Autodesk Fusion 360 part; units mm, degrees
sketch "Sketch1" plane through (0, 0, 0) normal (0, 1, 0) x (1, 0, 0)
  line L0 (-33.0001, 0) -> (-35.8285, -2.8284)
  line L1 (-33.0001, 0) -> (-33.002, 0) construction
  line L2 (-35.8285, -2.8284) -> (-35.8285, -23.8284)
  line L3 (-31.8323, -27.8284) -> (-31.8323, -32.0026)
  line L4 (-31.8323, -32.0026) -> (-59.8323, -32.0026)
  line L5 (-59.8323, -32.0026) -> (-59.8323, -48.0026)
  line L6 (-59.8323, -48.0026) -> (-31.8285, -48.0026)
  line L7 (-31.8285, -48.0026) -> (-31.8285, -50.0026)
  line L8 (-35.8285, -54.0026) -> (-35.8285, -75.0026)
  line L9 (-35.8285, -75.0026) -> (-33.0001, -77.8311)
  line L10 (-33.0001, -77.8311) -> (-1.0001, -77.8311)
  line L11 (-33.002, 0) -> (-1.002, 0)
  arc A0 (-35.8285, -54.0026) -> (-31.8285, -50.0026) centre (-35.8285, -50.0026) ccw
  arc A1 (-31.8323, -27.8284) -> (-35.8285, -23.8284) centre (-35.8323, -27.8284) ccw
  line L12 (-1.0001, -77.8311) -> (-1.002, 0)
  point P0 (-31.8323, -24.0026)
  point P1 (-31.8285, -54.0026)
  point P2 (-4.832, 0)
  dimension "d2" = 135
  dimension "d3" = 4
  dimension "d4" = 21
  dimension "d5" = 4
  dimension "d6" = 8
  dimension "d7" = 28
  dimension "d8" = 16
  dimension "d9" = 6
  dimension "d10" = 4
  dimension "d11" = 21
  dimension "d12" = 4
  dimension "d13" = 135
  dimension "d14" = 32
  dimension "d15" = 32
  dimension "d16" = 4
  dimension "d17" = 4
revolve "Revolve1" add sketch "Sketch1" angle 360 about axis through (0, 0, 1.75) along (0, 0, 1)
sketch "Sketch2" plane through (0, 0, 77.8311) normal (0, 0, 1) x (-1, 0, 0)
  circle A0 centre (0, 0) radius 1.0001
  circle A1 centre (0, 0) radius 33.0001
  circle A2 centre (0, 0) radius 24
  dimension "d19" = 48
extrude "Extrude1" cut sketch "Sketch2" against normal blind 110 contours A2
sketch "Sketch3" plane through (0, 0, 48.0026) normal (0, 0, 1) x (-1, 0, 0)
  circle A0 centre (0, 0) radius 31.8285
  circle A1 centre (0, 0) radius 59.8323
  circle A2 centre (0, 0) radius 54
  circle A3 centre (53.999, -0.3261) radius 4
  line L0 (0, 0) -> (27, -46.7654)
  line L1 (0, 0) -> (54, 0) construction
  circle A4 centre (27, -46.7654) radius 4
  line L2 (0, 0) -> (-27, -46.7654)
  line L3 (0, 0) -> (54, 0) construction
  circle A5 centre (-27, -46.7654) radius 4
  circle A6 centre (-54, 0) radius 4
  line L4 (0, 0) -> (-27, 46.7654)
  line L5 (0, 0) -> (54, 0) construction
  line L6 (0, 0) -> (27, 46.7654)
  line L7 (0, 0) -> (54, 0) construction
  circle A7 centre (27, 46.7654) radius 4
  circle A8 centre (-27, 46.7654) radius 4
  dimension "d22" = 108
  dimension "d23" = 8
  dimension "d24" = 60
  dimension "d25" = 8
  dimension "d26" = 120
  dimension "d27" = 8
  dimension "d28" = 8
  dimension "d29" = 120
  dimension "d30" = 60
  dimension "d31" = 54
  dimension "d32" = 8
  dimension "d33" = 8
hole "Hole1" at (-54, 0, 48.0026) at (-27, 46.7654, 48.0026) at (27, 46.7654, 48.0026) at (54, 0, 48.0026) at (27, -46.7654, 48.0026) at (-27, -46.7654, 48.0026) direction (0, 0, -1) diameter 6.78 depth 15 tip angle 118
extrude "Extrude2" [suppressed]
Can you work these out from the model? Positions are in its coordinate system, mm. A direction names the side the tool comes from. Give positions to 0.01 mm unless a question says otherwise; leave off trailing zeros. Order: outer loops, then holes, each group sorted by start corner. A loop starts at its lowest first (then second) coordinate and runs counter-clockwise, first axis right, second up. Notation, with made-up numbers: M -23,17.25 L 16,17.25 A22 ccw 16,38.25 Z; hole C 47.5,-19.5 d11. An arc over 180 degrees is marked long. Use a Markdown table: item, result. Add a question column.
Item 1: Suppose I cut it at B-B (x = 54). List the corners of the cut face in (y, z) for me, then the cut area to 3 significant figures.
Item 2: We'd pull the mould along Y, two halves only. Please class faces 4 (the cylindrical face through (50.64, 0.44, 40.4)), 5 (the cylindrical face through (31.798, -1.399, 49.017)), 6 (the flat face through (-26, 26, 32.003)): +Y half, -Y half, draft (parallel to the pull), parting line (faces both ways), or undercut.
Item 3: Suppose I cut it at C-C (z = 70.5). List the corners of the cut face in (x, y) for me.
Item 4: Suppose I cut it at A-A (z = 43.5). List the corners of the cut face in (x, y) for me.
Item 5: If I drill on L1, parallel to X at y = 0, z = 41; L2, parallel to Y at x = -1, z = 74; L3, parallel to Z at x = -29, y = -18, over which ranges is the centre line in solid material (lowest first)? Write a range as [from, to].
Item 6: For faces 1 (the cylindrical face through (25.982, 43.532, 40.398)), 2 (the cylindrical face through (7.767, 34.977, 13.475)), 3 (the cylindrical face through (6.901, 31.075, 29.945)), which set-ups out of +Z, -Z, +X, -X, +Y, -Y let a thin tool reach every point of the face, with its end or its side?
Item 7: Suppose I cut it at D-D (x = -27). Count the separate pieces of the cut face and the enclosed holes in it, then the cut area to 3 significant figures.
Item 8: Will these pins go through, and if not, where does the flat tip stop? pin 1 (1 mm diameter, centred on x = -45.5, y = 4, fed in from +Z); pin 2 (5.5 mm diameter, centred on x = 27, y = -46.77, fed in from -Z); pin 3 (6 mm diameter, centred on x = -54, y = 0, fed in from +Z).
Answer sheet:
| question | item | result |
|---|---|---|
| 1 | outline | M -25.77,32 L -1.73,32 L -3.39,33 L -3.39,48 L -25.77,48 Z; M 1.73,32 L 25.77,32 L 25.77,48 L 3.39,48 L 3.39,33 Z |
| 1 | area | 718 mm² |
| 2 | face 4 | undercut |
| 2 | face 5 | parting line |
| 2 | face 6 | draft |
| 3 | outline | C 0,0 d71.66; hole C 0,0 d48 |
| 4 | outline | C 0,0 d119.66; hole C -54,0 d6.78; hole C -27,-46.77 d6.78; hole C -27,46.77 d6.78; hole C 0,0 d48; hole C 27,-46.77 d6.78; hole C 27,46.77 d6.78; hole C 54,0 d6.78 |
| 5 | L1 | x = [-59.83, -57.39], [-50.61, -24], [24, 50.61], [57.39, 59.83] |
| 5 | L2 | y = [-35.81, -23.98], [23.98, 35.81] |
| 5 | L3 | z = [1.13, 24.21], [32, 48], [53.63, 76.7] |
| 6 | face 1 | +Z |
| 6 | face 2 | -Z |
| 6 | face 3 | none |
| 7 | separate pieces | 3 |
| 7 | enclosed holes | 0 |
| 7 | area | 4,220 mm² |
| 8 | pin 1 | stops at z = 48 |
| 8 | pin 2 | stops at z = 32 |
| 8 | pin 3 | stops at z = 32.77 |
